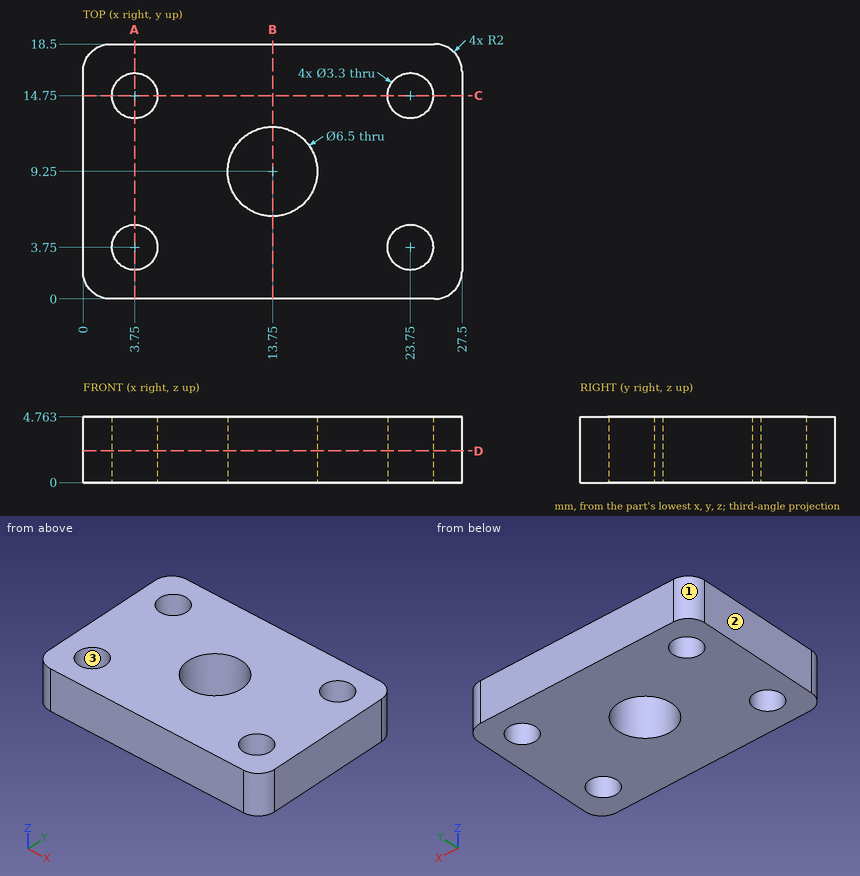
Can you work these out from the drawing? Everything is in mm from the part's minimum corner. Give positions to 0.01 mm unless a question says otherwise; leave off trailing zeros. Order: outer loops, then holes, each group sorted by start corner. A loop starts at its lowest first (then second) coordinate and runs counter-clockwise, first axis right, second up.
1. We'd pull the mould along Y, two halves only. Please class the marked faces 1, 2 and 3: pulls with the +Y half, pulls with the -Y half, needs draft (parallel to the pull), parting line crosses it, or undercut.
2. Suppose I cut it at D-D (z = 2.3). List the corners of the cut face in (x, y) for me, plus the area to 3 significant figures.
3. Suppose I cut it at A-A (x = 3.75). List the corners of the cut face in (y, z) for me.
4. I need wall thicknesses on L1, parallel to Y at x = 3.75, z = 3.15; L2, parallel to X at y = 14.75, z = 2.9; L3, parallel to Y at x = 13.75, z = 1.55. Which ranges of each line are inside material? Lowest first, please.
5. Suppose I cut it at C-C (y = 14.75). List the corners of the cut face in (x, z) for me.
6. Suppose I cut it at B-B (x = 13.75). List the corners of the cut face in (y, z) for me.
Solved:
1. face 1: pulls with the +Y half
1. face 2: needs draft
1. face 3: undercut
2. outline: (0, 2) arc R2 ccw to (2, 0) - (25.5, 0) arc R2 ccw to (27.5, 2) - (27.5, 16.5) arc R2 ccw to (25.5, 18.5) - (2, 18.5) arc R2 ccw to (0, 16.5) - close; hole circle Ø3.3 at (3.75, 3.75); hole circle Ø3.3 at (3.75, 14.75); hole circle Ø6.5 at (13.75, 9.25); hole circle Ø3.3 at (23.75, 3.75); hole circle Ø3.3 at (23.75, 14.75)
2. area: 438 mm2
3. outline: (0, 0) - (2.1, 0) - (2.1, 4.76) - (0, 4.76) - close; (5.4, 0) - (13.1, 0) - (13.1, 4.76) - (5.4, 4.76) - close; (16.4, 0) - (18.5, 0) - (18.5, 4.76) - (16.4, 4.76) - close
4. L1: y = 0 to 2.1, 5.4 to 13.1, 16.4 to 18.5
4. L2: x = 0 to 2.1, 5.4 to 22.1, 25.4 to 27.5
4. L3: y = 0 to 6, 12.5 to 18.5
5. outline: (0, 0) - (2.1, 0) - (2.1, 4.76) - (0, 4.76) - close; (5.4, 0) - (22.1, 0) - (22.1, 4.76) - (5.4, 4.76) - close; (25.4, 0) - (27.5, 0) - (27.5, 4.76) - (25.4, 4.76) - close
6. outline: (0, 0) - (6, 0) - (6, 4.76) - (0, 4.76) - close; (12.5, 0) - (18.5, 0) - (18.5, 4.76) - (12.5, 4.76) - close
